Build history of the part. All positions in model axes, mm. A direction names the side the tool comes from. Coordinates: 2 decimals unless noted, no trailing zeros. Loops run counter-clockwise (first coordinate to the right, second up) from the corner with the lowest first, then second, coordinate; pieces in that order, holes last.
(1) Slice it at A-A (z = -22). Give the cut face in (x, y), and give its area (3 significant figures).
(2) Slice it at B-B (y = -156.5). Give the cut face in (x, z).
(3) Two-plate mould, pull along X, no slides. Class faces 1 (the face through (50, 0, 1)), 2 (the face through (-76.675, -103, -1)), 3 (the face through (-1, -103, 40.285)), 4 (the face through (-1, -103, -40.285)): pulls with the +X half, pulls with the -X half, needs draft (parallel to the pull), parting line crosses it, or undercut.
(4) Slice it at C-C (x = -20). Give the cut face in (y, z), and give its area (3 significant figures).
(5) Wall check: L1, parallel to X at y = -108, z = 1.5; L2, parallel to Z at x = 43, y = -77. Give the ranges that are in metal, low to high.
(6) Tool access for faces 5 (the face through (-1, -103, 77.009)), 6 (the face through (-43.717, -103, -1)): list every direction of +Z, -Z, +X, -X, +Y, -Y with a clear straight run to the whole face (end or side of a thin tool).
from build123d import *

# Parameters (mm, degrees)
F0_W     = 153.35077
F0_H     = 154.018536
F0_W_2   = 87.434582
F0_H_2   = 80.570326
F1_DEPTH = 35
F2_DEPTH = 208


with BuildPart() as f1:
    # F0 (on Front) → F1 (new body)
    with BuildSketch(Plane.XZ):
        Rectangle(F0_W, F0_H)
        Rectangle(F0_W_2, F0_H_2, mode=Mode.SUBTRACT)
    extrude(amount=F1_DEPTH)

    # F0 (on Front) → F2 (join)
    with BuildSketch(Plane.XZ):
        Rectangle(F0_W, F0_H)
        Rectangle(F0_W_2, F0_H_2, mode=Mode.SUBTRACT)
    extrude(amount=F2_DEPTH)


solid = f1.part
Response values:
1. outline: (-76.68, -208) - (-43.72, -208) - (-43.72, 0) - (-76.68, 0) - close; (43.72, -208) - (76.68, -208) - (76.68, 0) - (43.72, 0) - close
1. area: 13,700 mm2
2. outline: (-76.68, -77.01) - (76.68, -77.01) - (76.68, 77.01) - (-76.68, 77.01) - close; hole (-43.72, -40.29) - (43.72, -40.29) - (43.72, 40.29) - (-43.72, 40.29) - close
3. face 1: needs draft
3. face 2: pulls with the -X half
3. face 3: undercut
3. face 4: undercut
4. outline: (-208, -77.01) - (0, -77.01) - (0, -40.29) - (-208, -40.29) - close; (-208, 40.29) - (0, 40.29) - (0, 77.01) - (-208, 77.01) - close
4. area: 15,300 mm2
5. L1: x = -76.68 to -43.72, 43.72 to 76.68
5. L2: z = -77.01 to -40.29, 40.29 to 77.01
6. face 5: +Z, +X, -X, +Y, -Y
6. face 6: +Y, -Y
